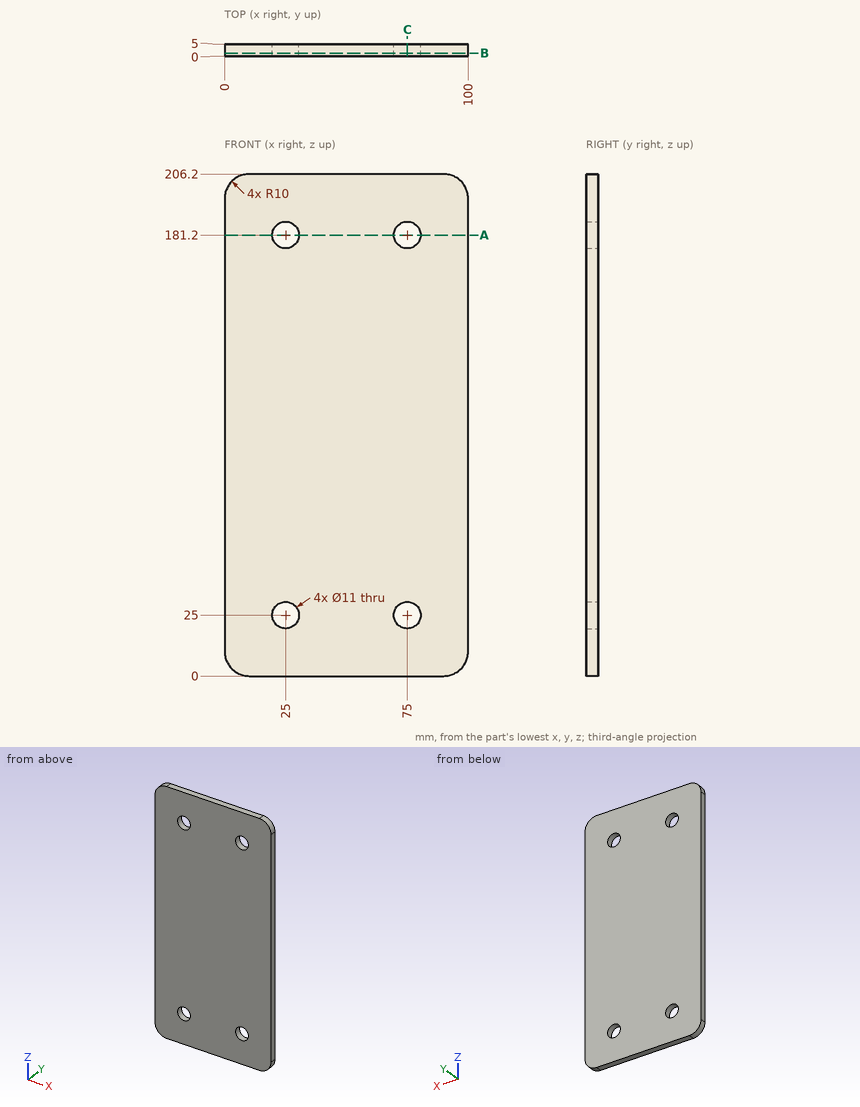
The drawing under review shows one solid part. Ordinate dimensions are in mm from its lowest x, y, z. Round coordinates to 2 decimals unless told otherwise and drop trailing zeros. Order: outer loops, then holes, each group sorted by start corner. A loop starts at its lowest first (then second) coordinate and runs counter-clockwise, first axis right, second up. Notation, with made-up numbers: M -32.5,-17.5 L 14.5,-17.5 A20 cw 14.5,15.5 Z; hole C 47,-24.75 d11. An arc over 180 degrees is marked long. Answer as CSV lines item,"result". Start each with the question number.
1) Add section C-C (x = 75). Give the boundary of the cut face in (y, z), then the cut area to 3 significant figures.
2) Add section A-A (z = 181.2). Give the boundary of the cut face in (x, y).
3) Wall thickness on line 1 along Z through (x, y) = (75, 1.05); line 2 along X through (y, z) = (3.15, 24.5); line 3 along Z through (x, y) = (27.5, 0.5): over which ranges is each line inside the solid? List them lowest first. Write a range as [from, to].
4) Add section B-B (y = 1.25). Give the boundary of the cut face in (x, z).
5) For pin 1 Ø3 at (x, y) = (55.5, 1) entering from -Z; pin 2 Ø9 at (x, z) = (75, 25) entering from -Y (1 decimal), all flat-tipped, find the tip position at first contact; note any pin that passes through.
Resolved:
1,outline,"M 0,0 L 5,0 L 5,19.5 L 0,19.5 Z; M 0,30.5 L 5,30.5 L 5,175.7 L 0,175.7 Z; M 0,186.7 L 5,186.7 L 5,206.2 L 0,206.2 Z"
1,area,"921 mm^2"
2,outline,"M 0,0 L 19.5,0 L 19.5,5 L 0,5 Z; M 30.5,0 L 69.5,0 L 69.5,5 L 30.5,5 Z; M 80.5,0 L 100,0 L 100,5 L 80.5,5 Z"
3,line 1,"[0, 19.5], [30.5, 175.7], [186.7, 206.2]"
3,line 2,"[0, 19.52], [30.48, 69.52], [80.48, 100]"
3,line 3,"[0, 20.1], [29.9, 176.3], [186.1, 206.2]"
4,outline,"M 0,10 A10 ccw 10,0 L 90,0 A10 ccw 100,10 L 100,196.2 A10 ccw 90,206.2 L 10,206.2 A10 ccw 0,196.2 Z; hole C 25,25 d11; hole C 25,181.2 d11; hole C 75,25 d11; hole C 75,181.2 d11"
5,pin 1,"z = 0"
5,pin 2,"through"
